```python
from build123d import *
from build123d.topology import SkipClean

# Parameters (mm, degrees)
ESQUISSE1_W                   = 100
ESQUISSE1_H                   = 102.5
ESQUISSE1_W_2                 = 80
ESQUISSE1_H_2                 = 82.5
BOSS_EXTRU_3_DEPTH            = 88
BOSS_EXTRU_4_DEPTH            = 102.5
ESQUISSE7_W                   = 40
ESQUISSE7_H                   = 40
ESQUISSE7_W_2                 = 20
ESQUISSE7_H_2                 = 20
BOSS_EXTRU_11_DEPTH           = 105.5
ENL_V_MAT_EXTRU_9_REACH       = 240.16
ESQUISSE13_W                  = 10
ESQUISSE13_H                  = 20
BOSS_EXTRU_12_DEPTH           = 2.5
ESQUISSE17_R                  = 5
ESQUISSE17_W                  = 40
ESQUISSE17_H                  = 20
BOSS_EXTRU_13_DEPTH           = 51.25
ENL_V_MAT_EXTRU_12_DEPTH      = 262.252326841
ENL_V_MAT_EXTRU_12_DEPTH_BACK = 262.252326841
ESQUISSE18_R                  = 5
ENL_V_MAT_EXTRU_13_REACH      = 234.659
ESQUISSE19_W                  = 10
ESQUISSE19_H                  = 20
CONG_1_R                      = 10
ENL_V_MAT_EXTRU_15_DEPTH      = 88


with BuildPart() as part:
    # Esquisse1 → Boss.-Extru.3 (new body)
    with BuildSketch(Plane(origin=(0, 0, 0), x_dir=(1, 0, 0), z_dir=(0, 1, 0))):
        Rectangle(ESQUISSE1_W, ESQUISSE1_H)
        Rectangle(ESQUISSE1_W_2, ESQUISSE1_H_2, mode=Mode.SUBTRACT)
    extrude(amount=BOSS_EXTRU_3_DEPTH)

    # Esquisse3 → Boss.-Extru.4 (add)
    with BuildSketch(Plane.XY.offset(51.25)):
        Polygon((50, 6), (50, 0), (96.658434537, 0), (130.222419784, 40), (190.222419784, 40), (190.222419784, 46), (127.424573836, 46), (93.860588588, 6), align=None)
    extrude(amount=-BOSS_EXTRU_4_DEPTH)

    # Esquisse7 → Boss.-Extru.11 (add)
    with BuildSketch(Plane.XZ.offset(-40)):
        with Locations((190.222419784, 0)):
            Rectangle(ESQUISSE7_W, ESQUISSE7_H)
        with Locations((190.222419784, 0)):
            Rectangle(ESQUISSE7_W_2, ESQUISSE7_H_2, mode=Mode.SUBTRACT)
    extrude(amount=-BOSS_EXTRU_11_DEPTH)

    # Esquisse13 → Enlèv. mat.-Extru.9 (cut, up to next)
    with BuildSketch(Plane(origin=(0, 46, 0), x_dir=(1, 0, 0), z_dir=(0, 1, 0)), mode=Mode.PRIVATE) as enl_v_mat_extru_9_sk1:
        with Locations((185.222419784, 0)):
            Rectangle(ESQUISSE13_W, ESQUISSE13_H)
    enl_v_mat_extru_9_tool1 = extrude(enl_v_mat_extru_9_sk1.sketch, amount=-ENL_V_MAT_EXTRU_9_REACH, mode=Mode.PRIVATE) & part.part
    add(enl_v_mat_extru_9_tool1.solids().sort_by_distance((185.22242, 46, 0))[0], mode=Mode.SUBTRACT)

    # Esquisse14 → Boss.-Extru.12 (add, symmetric)
    with BuildSketch(Plane.XY):
        Polygon((50, 88), (103.597078503, 88), (151.845307295, 145.5), (170.222419784, 145.5), (170.222419784, 46), (127.424573836, 46), (93.860588588, 6), (50, 6), align=None)
    extrude(amount=BOSS_EXTRU_12_DEPTH, both=True)

    # Esquisse17 → Boss.-Extru.13 (add, symmetric)
    # profile 1 of 2: a face of its own
    with BuildSketch(Plane.XY):
        Polygon((44, 20), (44, 0), (75, 0), (75, 6), (75, 20), align=None)
        with Locations((65, 10)):
            Circle(ESQUISSE17_R, mode=Mode.SUBTRACT)
    # profile 2 of 2: a face of its own
    with BuildSketch(Plane.XY):
        with Locations((170.222419784, 50)):
            Rectangle(ESQUISSE17_W, ESQUISSE17_H)
        with Locations((160.222419784, 50)):
            Circle(ESQUISSE17_R, mode=Mode.SUBTRACT)
    extrude(amount=BOSS_EXTRU_13_DEPTH, both=True)

    # Esquisse18 → Enlèv. mat.-Extru.12 (cut, two sides: drawn at the far end of the back side and taken through both)
    with SkipClean():  # the faces are left unmerged after this step: merging them gives an invalid solid
        with BuildSketch(Plane.XY.offset(2.5).offset(-ENL_V_MAT_EXTRU_12_DEPTH_BACK)):
            with Locations(Location((160.222419784, 50, 0), (0, 0, 180))):
                Circle(ESQUISSE18_R)
            with Locations(Location((65, 10, 0), (0, 0, 180))):
                Circle(ESQUISSE18_R)
        extrude(amount=ENL_V_MAT_EXTRU_12_DEPTH + ENL_V_MAT_EXTRU_12_DEPTH_BACK, mode=Mode.SUBTRACT)

    # Esquisse19 → Enlèv. mat.-Extru.13 (cut, up to next)
    with BuildSketch(Plane(origin=(0, 60, 0), x_dir=(1, 0, 0), z_dir=(0, 1, 0)), mode=Mode.PRIVATE) as enl_v_mat_extru_13_sk1:
        with Locations((185.222419784, 0)):
            Rectangle(ESQUISSE19_W, ESQUISSE19_H)
    enl_v_mat_extru_13_tool1 = extrude(enl_v_mat_extru_13_sk1.sketch, amount=-ENL_V_MAT_EXTRU_13_REACH, mode=Mode.PRIVATE) & part.part
    add(enl_v_mat_extru_13_tool1.solids().sort_by_distance((185.22242, 60, 0))[0], mode=Mode.SUBTRACT)

    # Congé1
    cong_1_edges = [part.edges().sort_by_distance(p)[0] for p in [
        (93.860588588, 6, 26.875),
        (127.424573836, 46, 26.875),
        (151.845307295, 145.5, 0),
        (103.597078503, 88, 0),
        (75, 20, 26.875),
        (75, 20, -26.875),
        (150.222419784, 60, 26.875),
        (150.222419784, 60, -26.875),
        (127.424573836, 46, -26.875),
        (93.860588588, 6, -26.875),
        (96.658434537, 0, 0),
        (130.222419784, 40, 0),
    ]]
    fillet(cong_1_edges, radius=CONG_1_R)

    # Esquisse20 → Enlèv. mat.-Extru.15 (cut)
    with SkipClean():  # the faces are left unmerged after this step: merging them gives an invalid solid
        with BuildSketch(Plane(origin=(0, 0, 0), x_dir=(1, 0, 0), z_dir=(0, 1, 0))):
            Polygon((6, 51.25), (190.222419784, 20), (210.222419784, 20), (210.222419784, 51.25), align=None)
            Polygon((210.222419784, -20), (190.222419784, -20), (6, -51.25), (210.222419784, -51.25), align=None)
        extrude(amount=ENL_V_MAT_EXTRU_15_DEPTH, mode=Mode.SUBTRACT)


solid = part.part
```
Can you work these out from the model? Positions are in its coordinate system, mm. A direction names the side the tool comes from. Round coordinates to 2 decimals unless told otherwise and drop trailing zeros. Loops run counter-clockwise (first coordinate to the right, second up) from the corner with the lowest first, then second, coordinate; pieces in that order, holes last. Notation, with made-up numbers: (67.5, -19.5) -> (104.5, -19.5) arc R9 ccw to (104.5, -15.5) -> close; hole circle Ø3 at (35.5, 1). An arc over 180 degrees is marked (long way). Answer in a Markdown table with one row per item.
Item 1: Suppose I cut it at A-A, the plane x = -10. List the corners of the cut face in (y, z) for me, plus the area to 3 significant figures.
Answer block:
| item | result |
|---|---|
| outline | (0, -51.25) -> (88, -51.25) -> (88, -41.25) -> (0, -41.25) -> close; (0, 41.25) -> (88, 41.25) -> (88, 51.25) -> (0, 51.25) -> close |
| area | 1,760 mm² |
Item 2: Will these pins go through, and if not, where does the flat tip stop? P1, Ø14.5, axis at x = 138.5, z = -17, coming from the +Y side; P2, Ø20, axis at x = 193.5, y = 79.5, coming from the -Z side; P3, Ø10, axis at x = 94, z = 17, coming from the -Y side; P4, Ø11.5, axis at x = 78.5, z = 25, coming from the +Y side.
Answer block:
| item | result |
|---|---|
| P1 | y = 46 |
| P2 | z = -20 |
| P3 | y = 0 |
| P4 | y = 16.32 |
Item 3: If I drill on probe 1 along X at (y, z) = (82, -2); probe 2 along X at (y, z) = (50, -11); probe 3 along X at (y, z) = (75.5, 3.5), over which ranges is the centre line in solid material (lowest first)?
Answer block:
| item | result |
|---|---|
| probe 1 | -50 to -40, 40 to 180.22, 200.22 to 210.22 |
| probe 2 | -50 to -40, 40 to 50, 150.22 to 155.22, 165.22 to 210.22 |
| probe 3 | -50 to -40, 40 to 50, 170.22 to 180.22, 200.22 to 210.22 |
Item 4: We'd pull the mould along Z, two halves only. Please class faces 5 (the flat face through (190, 93, -10)), 6 (the flat face through (190, 92, -20)), 7 (the flat face through (113.25, 19.77, 0.5)): released by +Z, released by -Z, zero draft, split by the parting line, or undercut.
Answer block:
| item | result |
|---|---|
| face 5 | undercut |
| face 6 | released by -Z |
| face 7 | zero draft |
Item 5: Suppose I cut it at B-B, the plane y = 85. List the corners of the cut face in (x, z) for me, plus the area to 3 significant figures.
Answer block:
| item | result |
|---|---|
| outline | (-50, -51.25) -> (6, -51.25) -> (50, -43.79) -> (50, -2.5) -> (170.22, -2.5) -> (170.22, -20) -> (210.22, -20) -> (210.22, 20) -> (170.22, 20) -> (170.22, 2.5) -> (50, 2.5) -> (50, 43.79) -> (6, 51.25) -> (-50, 51.25) -> close; hole (-40, -41.25) -> (40, -41.25) -> (40, 41.25) -> (-40, 41.25) -> close; hole (180.22, -10) -> (200.22, -10) -> (200.22, 10) -> (180.22, 10) -> close |
| area | 5,120 mm² |
Item 6: On a 3-axis mill with a long thin cutter (end or side, diameter ignored), from which of +Z, -Z, +X, -X, +Y, -Y can I reach the whole of each face in a straight line? I mean faces 1 (the cylindrical face through (127.92, 45.09, -17.03)), 2 (the flat face through (200.222, 92, 0)), 3 (the flat face through (164, 40, 0)), 4 (the cylindrical face through (127.81, 45.04, 16.63)). Say none if no direction works.
Answer block:
| item | result |
|---|---|
| face 1 | -Z, +Y |
| face 2 | +Y, -Y |
| face 3 | +Z, -Z, +X, -Y |
| face 4 | +Z, +Y |
Item 7: Suppose I cut it at C-C, the plane x = 33. List the corners of the cut face in (y, z) for me, plus the area to 3 significant figures.
Answer block:
| item | result |
|---|---|
| outline | (0, -46.67) -> (88, -46.67) -> (88, -41.25) -> (0, -41.25) -> close; (0, 41.25) -> (88, 41.25) -> (88, 46.67) -> (0, 46.67) -> close |
| area | 954 mm² |
